The figure shows three views and two pictorial views of one solid part (mm, origin at its lowest corner). Answer the questions. Round coordinates to 2 decimals unless told otherwise and drop trailing zeros. Loops run counter-clockwise (first coordinate to the right, second up) from the corner with the lowest first, then second, coordinate; pieces in that order, holes last. Notation, with made-up numbers: (-28, 39) -> (-15, 39) arc R22 ccw to (-15, 56) -> close; hole circle Ø3 at (18.25, 57.25). An arc over 180 degrees is marked (long way). Use a Markdown table: item, result. Add a question column.
Q1. Section A-A on y = 2.85 is taken. Give the vertices of the cut face in (x, z).
Q2. Consider line 1 (Z direction, x = 46, y = 2.8); line 2 (X direction, y = 0.8, z = 85); line 3 (X direction, y = 4.05, z = 42.5). Determine where each line is inside the solid, lowest interval first.
Q3. Section C-C on x = 44 is taken. Give the vertices of the cut face in (y, z).
Q4. Given pin 1 Ø2.5 at (y, z) = (2.5, 1.5) entering from +X; pin 2 Ø1.5 at (y, z) = (3, 90) entering from -X; pin 3 Ø2.5 at (x, y) = (42, 3) entering from -Z; pin 4 Ø1 at (y, z) = (4.5, 55.5) entering from -X, each flat-ended and moving along its own axis, determine where each tip first touches the part or whether it passes through.
Q5. Section B-B on z = 88.5 is taken. Give the vertices of the cut face in (x, y), then the cut area to 3 significant figures.
Q6. Section D-D on z = 34.5 is taken. Give the vertices of the cut face in (x, y) (1 decimal), then the cut area to 3 significant figures.
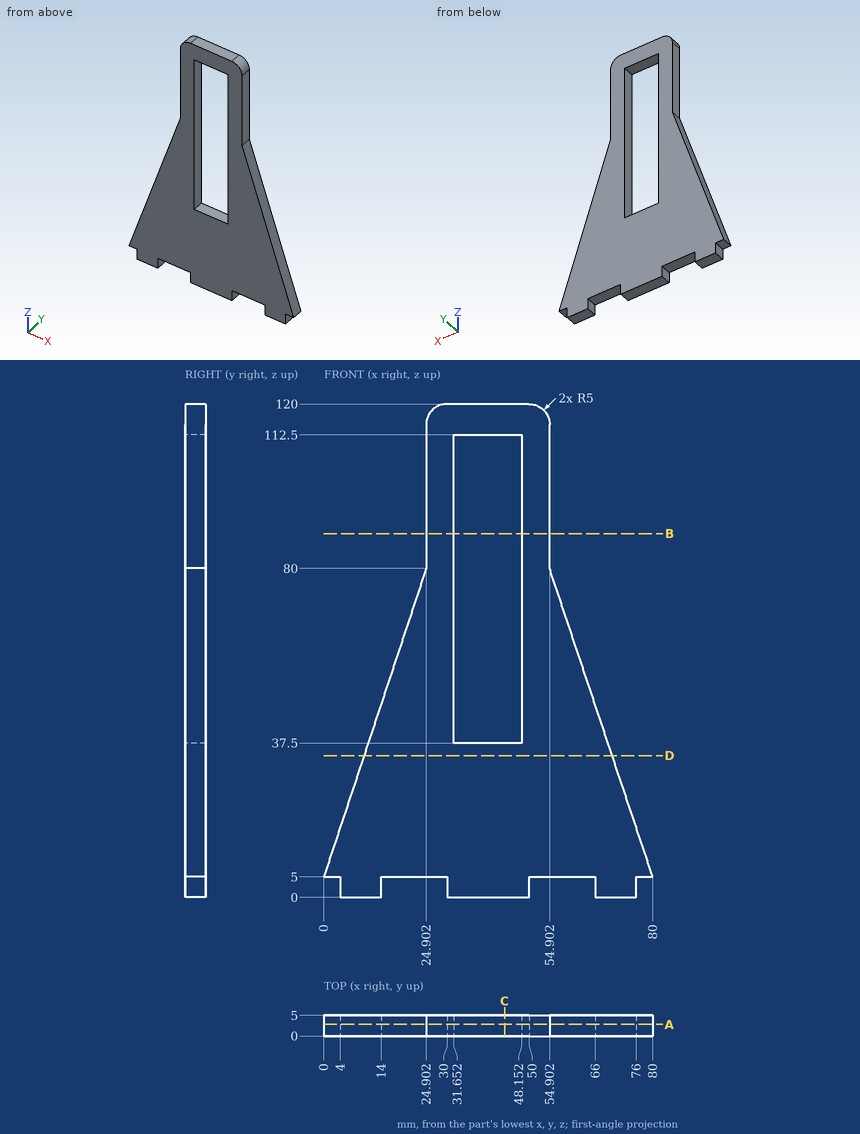
Checked values:
| question | item | result |
|---|---|---|
| 1 | outline | (0, 5) -> (4, 5) -> (4, 0) -> (14, 0) -> (14, 5) -> (30, 5) -> (30, 0) -> (50, 0) -> (50, 5) -> (66, 5) -> (66, 0) -> (76, 0) -> (76, 5) -> (80, 5) -> (54.9, 80) -> (54.9, 115) arc R5 ccw to (49.9, 120) -> (29.9, 120) arc R5 ccw to (24.9, 115) -> (24.9, 80) -> close; hole (31.65, 37.5) -> (48.15, 37.5) -> (48.15, 112.5) -> (31.65, 112.5) -> close |
| 2 | line 1 | z = 0 to 37.5, 112.5 to 120 |
| 2 | line 2 | x = 24.9 to 31.65, 48.15 to 54.9 |
| 2 | line 3 | x = 12.45 to 31.65, 48.15 to 67.45 |
| 3 | outline | (0, 0) -> (5, 0) -> (5, 37.5) -> (0, 37.5) -> close; (0, 112.5) -> (5, 112.5) -> (5, 120) -> (0, 120) -> close |
| 4 | pin 1 | stops at x = 76 |
| 4 | pin 2 | stops at x = 24.9 |
| 4 | pin 3 | stops at z = 0 |
| 4 | pin 4 | stops at x = 16.6 |
| 5 | outline | (24.9, 0) -> (31.65, 0) -> (31.65, 5) -> (24.9, 5) -> close; (48.15, 0) -> (54.9, 0) -> (54.9, 5) -> (48.15, 5) -> close |
| 5 | area | 67.5 mm2 |
| 6 | outline | (9.8, 0) -> (70.1, 0) -> (70.1, 5) -> (9.8, 5) -> close |
| 6 | area | 302 mm2 |
